Here's the drawing with two shaded views (mm, measured from the low corner). I have some questions. Round coordinates to 2 decimals unless told otherwise and drop trailing zeros. Order: outer loops, then holes, each group sorted by start corner. A loop starts at its lowest first (then second) coordinate and runs counter-clockwise, first axis right, second up. Notation, with made-up numbers: (23.25, 65.25) - (57.25, 65.25) arc R21 cw to (57.25, 93.25) - close; hole circle Ø10 at (-4, 85.5). An arc over 180 degrees is marked (long way). One line per item, written item: value.
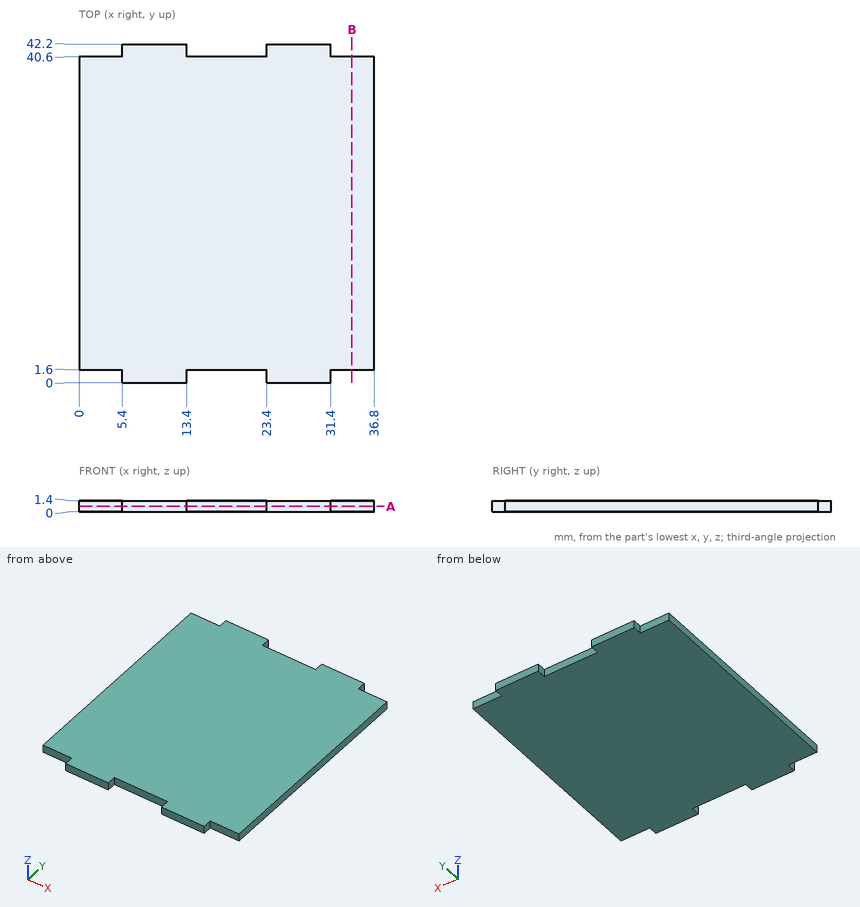
Q1. If I drill on line 1 along Y through (x, z) = (18, 0.1), over which ranges is the centre line in solid material (lowest first)?
Results list:
line 1: 1.6 to 40.6
Q2. If we section it at A-A, the plane z = 0.7: Please give me the cut outline in (x, y), then the cut area to 3 significant figures.
Results list:
outline: (0, 1.6) - (5.4, 1.6) - (5.4, 0) - (13.4, 0) - (13.4, 1.6) - (23.4, 1.6) - (23.4, 0) - (31.4, 0) - (31.4, 1.6) - (36.8, 1.6) - (36.8, 40.6) - (31.4, 40.6) - (31.4, 42.2) - (23.4, 42.2) - (23.4, 40.6) - (13.4, 40.6) - (13.4, 42.2) - (5.4, 42.2) - (5.4, 40.6) - (0, 40.6) - close
area: 1,490 mm²
Q3. If we section it at B-B, the plane x = 34: Please give me the cut outline in (y, z), then the cut area to 3 significant figures.
Results list:
outline: (1.6, 0) - (40.6, 0) - (40.6, 1.4) - (1.6, 1.4) - close
area: 54.6 mm²
Q4. Will these pins go through, and if not, where does the flat tip stop? pin 1 (0.7 mm diameter, centred on x = 4, z = 0.5, fed in from -Y); pin 2 (6 mm diameter, centred on x = 32.5, y = 24.5, fed in from -Z).
Results list:
pin 1: y = 1.6
pin 2: z = 0
